Job drawing, mm, ordinate dimensions from the low corner. One solid piece. Coordinates: 2 decimals unless noted, no trailing zeros. Write each loop counter-clockwise with the first axis right and the second up, starting at its lowest first coordinate (ties: lowest second). Pieces come first, ordered by that corner, then holes.
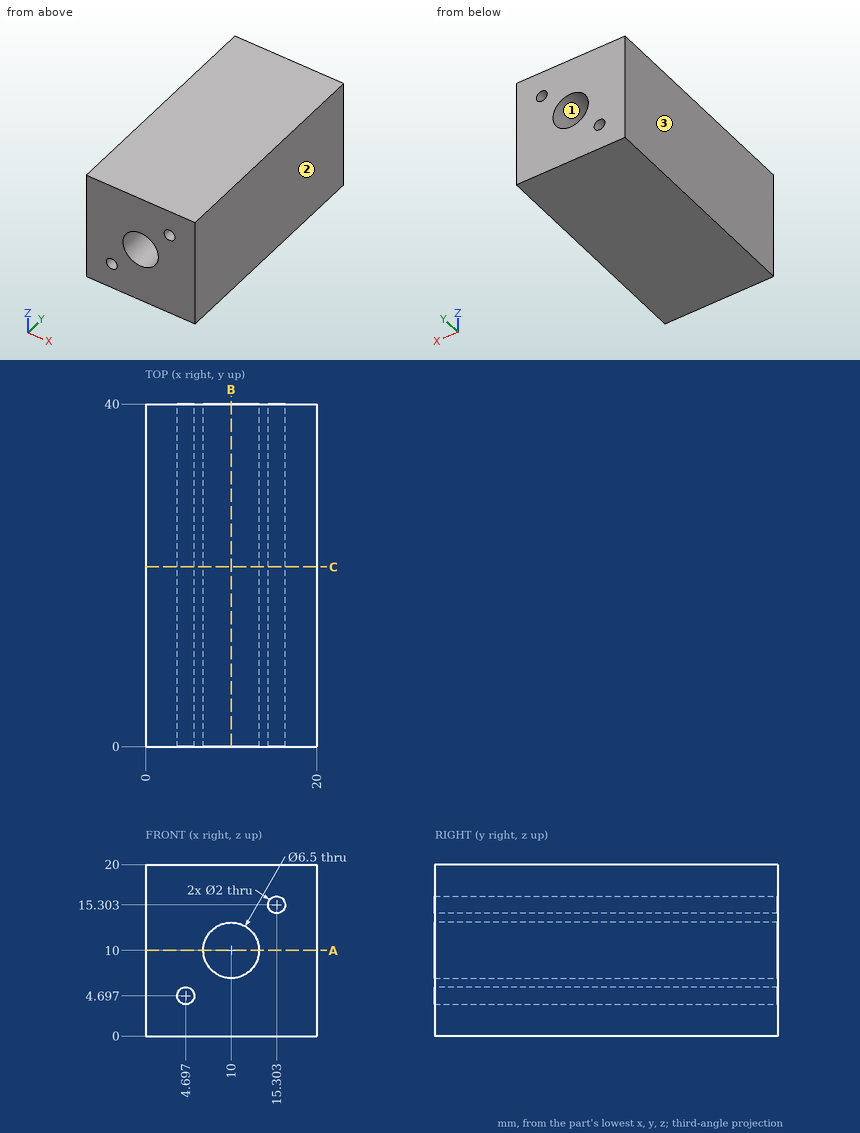
1. Mould opens along X. For the marked faces 1, 2 and 3 say: +X half, -X half, draft (parallel to the pull), parting line (faces both ways), or undercut.
Computed values:
face 1: undercut
face 2: +X half
face 3: -X half
2. Saw through at B-B on x = 10. List the corners of the cut face in (y, z), plus the area to 3 significant figures.
Computed values:
outline: (0, 0) - (40, 0) - (40, 6.75) - (0, 6.75) - close; (0, 13.25) - (40, 13.25) - (40, 20) - (0, 20) - close
area: 540 mm2
3. Saw through at A-A on z = 10. List the corners of the cut face in (x, y).
Computed values:
outline: (0, 0) - (6.75, 0) - (6.75, 40) - (0, 40) - close; (13.25, 0) - (20, 0) - (20, 40) - (13.25, 40) - close
4. Saw through at C-C on y = 21. List the corners of the cut face in (x, z).
Computed values:
outline: (0, 0) - (20, 0) - (20, 20) - (0, 20) - close; hole circle Ø2 at (4.7, 4.7); hole circle Ø6.5 at (10, 10); hole circle Ø2 at (15.3, 15.3)
5. Probe line 1 along Z through (x, y) = (10.25, 38.5); line 2 along Z through (x, y) = (15.5, 25.5); line 3 along X through (y, z) = (4.5, 12.5) (1 decimal). List the from-to ranges inside material, lowest first.
Computed values:
line 1: z = 0 to 6.76, 13.24 to 20
line 2: z = 0 to 14.32, 16.28 to 20
line 3: x = 0 to 7.9, 12.1 to 20
6. Flat gauge pin, fed straight in: pin 1 (5 mm diameter, centred on x = 10, z = 10, fed in from +Y). Where does the tip first touch, or does it go through?
Computed values:
pin 1: passes through
